```python
from build123d import *

# Parameters (mm, degrees)
SKETCH1_W           = 270
SKETCH1_H           = 110
BOSS_EXTRUDE1_DEPTH = 2
SKETCH5_R           = 1.5
CUT_EXTRUDE3_DEPTH  = 146.787516612
SKETCH6_R           = 1.6
CUT_EXTRUDE4_DEPTH  = 146.787516612
SKETCH7_R           = 3
CUT_EXTRUDE5_DEPTH  = 10
SKETCH8_R           = 30
SKETCH8_W           = 65
SKETCH8_H           = 20
CUT_EXTRUDE6_DEPTH  = 10


with BuildPart() as part:
    # Sketch1 → Boss-Extrude1 (new body)
    with BuildSketch(Plane.XY):
        Rectangle(SKETCH1_W, SKETCH1_H)
    extrude(amount=BOSS_EXTRUDE1_DEPTH)

    # Sketch5 → Cut-Extrude3 (cut, through all)
    with BuildSketch(Plane.XY.offset(2)):
        with Locations((-46.5, 24.75)):
            Circle(SKETCH5_R)
        with Locations((46.5, 24.75)):
            Circle(SKETCH5_R)
        with Locations((46.5, -24.75)):
            Circle(SKETCH5_R)
        with Locations((-46.5, -24.75)):
            Circle(SKETCH5_R)
    extrude(amount=-CUT_EXTRUDE3_DEPTH, mode=Mode.SUBTRACT)

    # Sketch6 → Cut-Extrude4 (cut, through all)
    with BuildSketch(Plane.XY.offset(2)):
        with Locations((-24, 15.549418684)):
            Circle(SKETCH6_R)
        with Locations((-30.4, 15.549418684)):
            Circle(SKETCH6_R)
        with Locations((-36.8, 15.549418684)):
            Circle(SKETCH6_R)
        with Locations((-43.2, 15.549418684)):
            Circle(SKETCH6_R)
        with Locations((-49.6, 15.549418684)):
            Circle(SKETCH6_R)
        with Locations((-56, 15.549418684)):
            Circle(SKETCH6_R)
        with Locations((-62.4, 15.549418684)):
            Circle(SKETCH6_R)
        with Locations((-62.4, -15.650581316)):
            Circle(SKETCH6_R)
        with Locations((-56, -15.650581316)):
            Circle(SKETCH6_R)
        with Locations((-49.6, -15.650581316)):
            Circle(SKETCH6_R)
        with Locations((-43.2, -15.650581316)):
            Circle(SKETCH6_R)
        with Locations((-36.8, -15.650581316)):
            Circle(SKETCH6_R)
        with Locations((-30.4, -15.650581316)):
            Circle(SKETCH6_R)
        with Locations((-24, -15.650581316)):
            Circle(SKETCH6_R)
        with Locations(Location((24, -15.650581316, 0), (0, 0, 180))):
            Circle(SKETCH6_R)
        with Locations(Location((30.4, -15.650581316, 0), (0, 0, 180))):
            Circle(SKETCH6_R)
        with Locations(Location((36.8, -15.650581316, 0), (0, 0, 180))):
            Circle(SKETCH6_R)
        with Locations(Location((43.2, -15.650581316, 0), (0, 0, 180))):
            Circle(SKETCH6_R)
        with Locations(Location((49.6, -15.650581316, 0), (0, 0, 180))):
            Circle(SKETCH6_R)
        with Locations(Location((56, -15.650581316, 0), (0, 0, 180))):
            Circle(SKETCH6_R)
        with Locations(Location((62.4, -15.650581316, 0), (0, 0, 180))):
            Circle(SKETCH6_R)
        with Locations(Location((62.4, 15.549418684, 0), (0, 0, 180))):
            Circle(SKETCH6_R)
        with Locations(Location((56, 15.549418684, 0), (0, 0, 180))):
            Circle(SKETCH6_R)
        with Locations(Location((49.6, 15.549418684, 0), (0, 0, 180))):
            Circle(SKETCH6_R)
        with Locations(Location((43.2, 15.549418684, 0), (0, 0, 180))):
            Circle(SKETCH6_R)
        with Locations(Location((36.8, 15.549418684, 0), (0, 0, 180))):
            Circle(SKETCH6_R)
        with Locations(Location((30.4, 15.549418684, 0), (0, 0, 180))):
            Circle(SKETCH6_R)
        with Locations(Location((24, 15.549418684, 0), (0, 0, 180))):
            Circle(SKETCH6_R)
    extrude(amount=-CUT_EXTRUDE4_DEPTH, mode=Mode.SUBTRACT)

    # Sketch7 → Cut-Extrude5 (cut)
    with BuildSketch(Plane(origin=(0, 0, 0), x_dir=(-1, 0, 0), z_dir=(0, 0, -1))):
        with Locations((-120, 46)):
            Circle(SKETCH7_R)
        with Locations((127, -46)):
            Circle(SKETCH7_R)
        with Locations((120, 46)):
            Circle(SKETCH7_R)
        with Locations((-127, -46)):
            Circle(SKETCH7_R)
    extrude(amount=-CUT_EXTRUDE5_DEPTH, mode=Mode.SUBTRACT)

    # Sketch8 → Cut-Extrude6 (cut)
    with BuildSketch(Plane(origin=(0, 0, 0), x_dir=(-1, 0, 0), z_dir=(0, 0, -1))):
        with Locations((94, 75)):
            Circle(SKETCH8_R)
        with Locations((-80.5, 45)):
            Rectangle(SKETCH8_W, SKETCH8_H)
    extrude(amount=-CUT_EXTRUDE6_DEPTH, mode=Mode.SUBTRACT)


solid = part.part
```
Input: part model. Units: mm. Frame: model coordinates. Round coordinates to 2 decimals unless told otherwise and drop trailing zeros. Loops run counter-clockwise (first coordinate to the right, second up) from the corner with the lowest first, then second, coordinate; pieces in that order, holes last. Notation, with made-up numbers: (53.25, 35) -> (102.25, 35) arc R23 ccw to (102.25, 69) -> close; hole circle Ø9 at (16, 84.25). An arc over 180 degrees is marked (long way). One line per item, written item: value.
(1) Section B-B (z = 1.6). Give the number of separate pieces and of enclosed holes in the cut face, plus the area to 3 significant figures.
Geometry check:
separate pieces: 1
enclosed holes: 36
area: 27,700 mm2
(2) Material intervals for line 1 (Y direction, x = -46.5, z = 1.35); line 2 (X direction, y = -45.5, z = 1.1); line 3 (Y direction, x = -30.4, z = 0.9), sorted ascending. Write a range as [from, to].
Geometry check:
line 1: [-55, -26.25], [-23.25, 23.25], [26.25, 55]
line 2: [-135, -129.96], [-124.04, 124.04], [129.96, 135]
line 3: [-55, -17.25], [-14.05, 13.95], [17.15, 55]
(3) Pin query (flat end, axial travel): pin 1 (3 mm diameter, centred on x = 49.6, y = -15.65, fed in from +Z); pin 2 (1 mm diameter, centred on x = 64.5, z = 0, fed in from +Y). Return the tip coordinate at first contact, or that it passes through.
Geometry check:
pin 1: through
pin 2: y = 35
(4) Section A-A (x = 120). Return the cut outline in (y, z), plus the area to 3 significant figures.
Geometry check:
outline: (-55, 0) -> (43, 0) -> (43, 2) -> (-55, 2) -> close; (49, 0) -> (55, 0) -> (55, 2) -> (49, 2) -> close
area: 208 mm2
